Build history of the part. All positions in model axes, mm. A direction names the side the tool comes from. Give positions to 0.01 mm unless a question says otherwise; leave off trailing zeros. Loops run counter-clockwise (first coordinate to the right, second up) from the corner with the lowest first, then second, coordinate; pieces in that order, holes last. Notation, with made-up numbers: M 62,22 L 96,22 A22 cw 96,28 Z; hole C 13.25,74.25 d3. An arc over 180 degrees is marked long. Answer as a JSON object with one key per item and string values. Group by question number.
1. Slice it at D-D (y = -22). List the corners of the cut face in (x, z) (3 decimals), then the cut area to 3 significant figures.
2. Slice it at A-A (x = 17.5). List the corners of the cut face in (y, z).
3. Drop flat-ended pins along their axis: pin 1 Ø3 at (x, z) = (-3, 23.5) entering from +Y; pin 2 Ø2.5 at (x, y) = (-12.5, 8.5) entering from -Z; pin 3 Ø6 at (y, z) = (-20, 15) entering from +X (3 decimals). Give the stop position or say it passes through.
4. Drill centre lines: line 1 along Y through (x, z) = (11.5, 18); line 2 along Y through (x, z) = (19, 11); line 3 along X through (y, z) = (-30, 24.25) (3 decimals). Where is each one in solid material? Low to high. Write a range as [from, to].
5. Mould opens along Y. For faces 1 (the face through (13.7, -21.8, 17.7)), 2 (the face through (13.7, -36.28, 12.88)), 3 (the face through (-25.4, 3, 13)) say: released by +Y, released by -Y, zero draft, split by the parting line, or undercut.
6. Slice it at B-B (z = 5). List the corners of the cut face in (x, y) (3 decimals).
7. Slice it at C-C (y = -0.5). List the corners of the cut face in (x, z) (3 decimals).
8. 3-axis set-ups, long thin cutter, end or side, ignore diameter. For faces 4 (the face through (5.491, -4.528, 9.798)), 5 (the face through (19.685, -22, 10)), 6 (the face through (-10, -4.91, 13)), 7 (the face through (13.72, -21.63, 0.36)): which of +Z, -Z, +X, -X, +Y, -Y reach the whole face in a straight line?
from build123d import *

# Parameters (mm, degrees)
F1_DEPTH = 26.67
F2_W     = 13.335
F2_H     = 6.35
F3_DEPTH = 16.51
F4_W     = 25.4
F4_H     = 13.3375799713
F5_DEPTH = 2.3241
F6_R     = 2.0701
F7_DEPTH = 21.9202
F8_R     = 1.27


with BuildPart() as f1:
    # F0 (on Top) → F1 (new body)
    with BuildSketch(Plane.XY):
        Polygon((19.685, 1.4401404459), (13.335, 1.4401404459), (13.335, -3.6108427172), (13.335, -4.9098595541), (13.335, -36.6598595541), (19.685, -36.6598595541), align=None)
        Polygon((13.335, -3.6108427172), (13.335, 1.4401404459), (0, 1.4401404459), (0, -4.9098595541), (13.335, -4.9098595541), align=None)
        Polygon((0, -4.9098595541), (0, 1.4401404459), (0, 6.9011404459), (-25.4, 6.9011404459), (-25.4, -4.9098595541), align=None)
    extrude(amount=F1_DEPTH)

    # F2 (on face) → F3 (cut)
    with BuildSketch(Plane.XY.offset(26.67)):
        with Locations((6.6675, -1.7348595541)):
            Rectangle(F2_W, F2_H)
        Polygon((19.685, 1.4401404459), (13.335, 1.4401404459), (13.335, -4.9098595541), (13.335, -21.4198595541), (19.685, -21.4198595541), align=None)
    extrude(amount=-F3_DEPTH, mode=Mode.SUBTRACT)

    # F4 (on face) → F5 (join)
    with BuildSketch(Plane(origin=(0, 6.9011404459, 0), x_dir=(-1, 0, 0), z_dir=(0, 1, 0))):
        with Locations((12.7, 20.0012100144)):
            Rectangle(F4_W, F4_H)
    extrude(amount=F5_DEPTH)

    # F6 (on face) → F7 (join, through all)
    with BuildSketch(Plane.YZ):
        with Locations((7.1678404459, 17.78)):
            Circle(F6_R)
    extrude(amount=F7_DEPTH)

    # F8
    f8_edges = [f1.edges().sort_by_distance(p)[0] for p in [
        (-6.0325, -4.90986, 0),
        (13.335, -4.90986, 5.08),
        (6.6675, -4.90986, 10.16),
        (0, -4.90986, 18.415),
        (-12.7, -4.90986, 26.67),
        (-25.4, -4.90986, 13.335),
        (13.335, -20.78486, 0),
        (13.335, -36.65986, 13.335),
        (13.335, -29.03986, 26.67),
        (13.335, -21.41986, 18.415),
        (13.335, -13.16486, 10.16),
        (-25.4, 2.15769, 26.67),
        (16.51, -36.65986, 26.67),
    ]]
    fillet(f8_edges, radius=F8_R)


solid = f1.part
Established:
{
 "1": {"outline": "M 13.335,1.27 A1.27 ccw 14.605,0 L 19.685,0 L 19.685,26.67 L 14.605,26.67 A1.27 ccw 13.539,26.09 L 13.539,9.58 A1.27 ccw 13.335,8.89 Z", "area": "165 mm^2"},
 "2": {"outline": "M -36.66,0 L 1.44,0 L 1.44,10.16 L -21.42,10.16 L -21.42,26.67 L -35.39,26.67 A1.27 ccw -36.66,25.4 Z; C 7.17,17.78 d4.14"},
 "3": {"pin 1": "stops at y = 9.23", "pin 2": "stops at z = 13.33", "pin 3": "stops at x = 19.685"},
 "4": {"line 1": "y = [5.11, 9.23]", "line 2": "y = [-36.66, -21.42]", "line 3": "x = [13.335, 19.685]"},
 "5": {"face 1": "undercut", "face 2": "released by -Y", "face 3": "zero draft"},
 "6": {"outline": "M -25.4,-3.64 A1.27 ccw -24.13,-4.91 L 12.065,-4.91 A1.27 cw 13.335,-6.18 L 13.335,-35.39 A1.27 ccw 14.605,-36.66 L 19.685,-36.66 L 19.685,1.44 L 0,1.44 L 0,6.901 L -25.4,6.901 Z"},
 "7": {"outline": "M -25.4,0 L 19.685,0 L 19.685,10.16 L 0,10.16 L 0,26.67 L -24.13,26.67 A1.27 ccw -25.4,25.4 Z"},
 "8": {"face 4": "+Z, -Y", "face 5": "+Z, -Z, +X, -Y", "face 6": "+Z, -Z, -X, -Y", "face 7": "-Z, -X, -Y"}
}
